The listing builds one solid part. Answer for the finished solid, in the listing's coordinates (mm). Face numbers are marked on the shaded views. A direction names the side the tool comes from. Round coordinates to 2 decimals unless told otherwise and drop trailing zeros. Order: outer loops, then holes, each group sorted by start corner. A loop starts at its lowest first (then second) coordinate and runs counter-clockwise, first axis right, second up. Notation, with made-up numbers: (-40, -27) -> (10, -27) arc R14 cw to (10, -1) -> close; hole circle Ø2 at (55, 28.25). An arc over 180 degrees is marked (long way). Return JSON: item names as keys, results as strings. Group by question number.
(1) Each of these flat-tipped pins is pushed along its axis until it touches: pin 1 (3 mm diameter, centred on x = -3, z = -36, fed in from -Y); pin 2 (1.5 mm diameter, centred on x = -8.5, y = -54, fed in from -Z); pin 3 (1.5 mm diameter, centred on x = -16.5, y = -109, fed in from -Z). Where does it stop, or does it pass through?
(2) Determine the mould class of the marked faces 1, 2 and 3 for opening direction Z: +Z half, -Z half, draft (parallel to the pull), parting line (faces both ways), or undercut.
(3) The part is cut by section A-A (z = -43.5). Determine the outline of the cut face in (x, y).
(4) The part is cut by section B-B (y = -66). Determine the outline of the cut face in (x, z), plus the area to 3 significant figures.
(5) Consider line 1 (Z direction, x = -11, y = -30); line 2 (Z direction, x = -12, y = -86.5); line 3 (X direction, y = -15.5, z = -11). Determine where each line is inside the solid, lowest interval first. Write a range as [from, to].
(6) The part is cut by section C-C (x = -19). Determine the outline of the cut face in (y, z), plus the area to 3 significant figures.
(7) The part is cut by section D-D (z = -15). Determine the outline of the cut face in (x, y), plus the area to 3 significant figures.
(8) Which of the six approach directions +Z, -Z, +X, -X, +Y, -Y give full straight-line access (tool end or side, diameter ignored) to the marked faces 4 and 5?
from build123d import *

# Parameters (mm, degrees)
SKETCH1_W           = 30
SKETCH1_H           = 80
BOSS_EXTRUDE1_DEPTH = 10
BOSS_EXTRUDE2_DEPTH = 80
FILLET1_R           = 10
FILLET2_R           = 10
FILLET4_R           = 10
SKETCH3_R           = 7.5
BOSS_EXTRUDE3_DEPTH = 150


with BuildPart() as part:
    # Sketch1 → Boss-Extrude1 (new body)
    with BuildSketch(Plane(origin=(0, 0, 0), x_dir=(1, 0, 0), z_dir=(0, 1, 0))):
        with Locations((-15, 40)):
            Rectangle(SKETCH1_W, SKETCH1_H)
    extrude(amount=BOSS_EXTRUDE1_DEPTH)

    # Sketch2 → Boss-Extrude2 (add)
    with BuildSketch(Plane(origin=(0, 0, -80), x_dir=(-1, 0, 0), z_dir=(0, 0, -1))):
        with BuildLine():
            Line((0, 10), (0, 35))
            Line((0, 35), (10, 60))
            ThreePointArc((10, 60), (13.809664499, 56.817288145), (15.008386018, 52))
            Line((15.008386018, 52), (30, 10))
            Line((30, 10), (30, 0))
            Line((30, 0), (0, 0))
            Line((0, 0), (0, 10))
        make_face()
    extrude(amount=-BOSS_EXTRUDE2_DEPTH)

    # Fillet1
    fillet1_edges = [part.edges().sort_by_distance(p)[0] for p in [
        (0, 35, -40),
    ]]
    fillet(fillet1_edges, radius=FILLET1_R)

    # Fillet2
    fillet2_edges = [part.edges().sort_by_distance(p)[0] for p in [
        (-15.008386018, 52, -40),
    ]]
    fillet(fillet2_edges, radius=FILLET2_R)

    # Fillet4
    fillet4_edges = [part.edges().sort_by_distance(p)[0] for p in [
        (-30, 10, -40),
    ]]
    fillet(fillet4_edges, radius=FILLET4_R)

    # Sketch3 → Boss-Extrude3 (add)
    with BuildSketch(Plane.XZ):
        with Locations(Location((-15, -15, 0), (0, 0, 90))):
            Circle(SKETCH3_R)
        with Locations(Location((-15, -65, 0), (0, 0, 90))):
            Circle(SKETCH3_R)
    extrude(amount=BOSS_EXTRUDE3_DEPTH)


solid = part.part
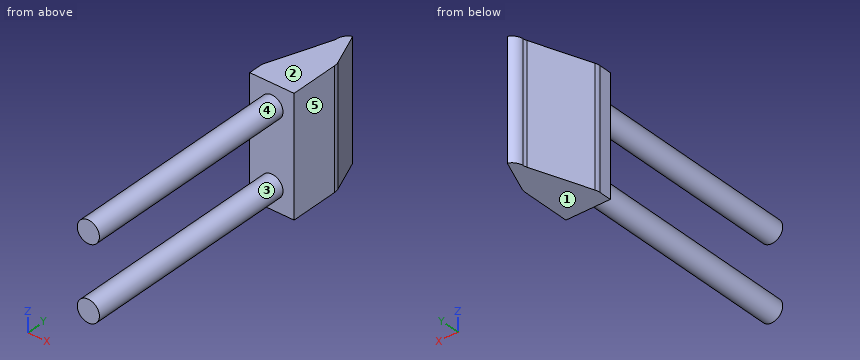
Answer below:
{
 "1": {"pin 1": "stops at y = 0", "pin 2": "stops at z = -69.82", "pin 3": "stops at z = -72.46"},
 "2": {"face 1": "-Z half", "face 2": "+Z half", "face 3": "undercut"},
 "3": {"outline": "(-30, 0) -> (0, 0) -> (0, 33.07) arc R10 ccw to (-0.72, 36.79) -> (-10, 60) arc R8 ccw to (-15.01, 53.11) arc R10 cw to (-15.57, 50.43) -> (-29.42, 11.63) arc R10 ccw to (-30, 8.27) -> close"},
 "4": {"outline": "circle Ø15 at (-15, -65); circle Ø15 at (-15, -15)", "area": "353 mm²"},
 "5": {"line 1": "z = [-71.34, -58.66], [-21.34, -8.66]", "line 2": "z = [-71.87, -58.13], [-21.87, -8.13]", "line 3": "x = [-21.34, -8.66]"},
 "6": {"outline": "(-150, -71.34) -> (0, -71.34) -> (0, -80) -> (40.82, -80) -> (40.82, 0) -> (0, 0) -> (0, -8.66) -> (-150, -8.66) -> (-150, -21.34) -> (0, -21.34) -> (0, -58.66) -> (-150, -58.66) -> close", "area": "7,070 mm²"},
 "7": {"outline": "(-30, 0) -> (-22.5, 0) -> (-22.5, -150) -> (-7.5, -150) -> (-7.5, 0) -> (0, 0) -> (0, 33.07) arc R10 ccw to (-0.72, 36.79) -> (-10, 60) arc R8 ccw to (-15.01, 53.11) arc R10 cw to (-15.57, 50.43) -> (-29.42, 11.63) arc R10 ccw to (-30, 8.27) -> close", "area": "3,480 mm²"},
 "8": {"face 4": "-Y", "face 5": "+Z, -Z, +X, +Y, -Y"}
}
